Verification items for the finished model (mm, model axes). A direction names the side the tool comes from. Coordinates: 2 decimals unless noted, no trailing zeros. Order: outer loops, then holes, each group sorted by start corner. A loop starts at its lowest first (then second) coordinate and runs counter-clockwise, first axis right, second up.
Q1. Set-up check for faces 1 (the flat face through (63.3, 50.6, 1.6)), 2 (the flat face through (49.9, 62.6, 1.6)), 3 (the flat face through (-62.6, 49.9, 1.6)): record each of +Z, -Z, +X, -X, +Y, -Y from which the full face is reachable in a straight line by a thin tool's end or side.
Q2. Depth check by flat-ended pin: P1, Ø1.5, axis at x = 65, z = 2, coming from the +Y side; P2, Ø1.5, axis at x = -42, z = 2, coming from the -Y side; P3, Ø1, axis at y = -24.5, z = 2.5, coming from the -X side. Enter the tip coordinate at first touch or a pass-through.
Q3. Cross-section at B-B, the plane y = 51.5. Record the boundary of the cut face in (x, z) (3 decimals), and give its area (3 significant figures).
Q4. Draft check along Y on faces 4 (the flat face through (-49.9, -62.6, 1.6)), 5 (the cylindrical face through (-0.419, 28.484, 1.565)), 6 (the flat face through (62.6, -49.9, 1.6)). Enter one of: pulls with the +Y half, pulls with the -Y half, needs draft (parallel to the pull), parting line crosses it, or undercut.
Q5. Cross-section at A-A, the plane x = -69. Record the boundary of the cut face in (y, z) (3 decimals), and give its area (3 significant figures).
Q6. Cross-section at D-D, the plane y = 12. Record the boundary of the cut face in (x, z) (3 decimals).
Q7. Thickness scan on line 1 (X direction, y = 59, z = 1.7); line 2 (Y direction, x = 74, z = 2.5); line 3 (X direction, y = -53.5, z = 1.85). Record the ranges inside material, lowest first.
from build123d import *

# Parameters (mm, degrees)
F0_W     = 177.8
F0_H     = 177.8
F1_DEPTH = 3.175
F3_DEPTH = 3.176
F4_R     = 38.1
F5_R     = 8.89


# Not quite as in the source:
# - a length typed as a fraction of an inch, garbled in the dataset ("3 / 203.2 mm" for 3/8 in), is restored


with BuildPart() as f1:
    # F0 (on Top) → F1 (new body)
    with BuildSketch(Plane.XY):
        Rectangle(F0_W, F0_H)
    extrude(amount=F1_DEPTH)

    # F2 (on face) → F3 (cut, through all)
    with BuildSketch(Plane.XY.offset(3.175)):
        Polygon((76.2, 88.9), (-76.2, 88.9), (0, 12.7), align=None)
        Polygon((88.9, -76.2), (88.9, 76.2), (12.7, 0), align=None)
        Polygon((-76.2, -88.9), (76.2, -88.9), (0, -12.7), align=None)
        Polygon((-12.7, 0), (-88.9, 76.2), (-88.9, -76.2), align=None)
    extrude(amount=-F3_DEPTH, mode=Mode.SUBTRACT)

    # F4
    f4_edges = [f1.edges().sort_by_distance(p)[0] for p in [
        (0, -12.7, 1.5875),
        (12.7, 0, 1.5875),
        (0, 12.7, 1.5875),
        (-12.7, 0, 1.5875),
    ]]
    fillet(f4_edges, radius=F4_R)

    # F5
    f5_edges = [f1.edges().sort_by_distance(p)[0] for p in [
        (88.9, 88.9, 1.5875),
        (88.9, 76.2, 1.5875),
        (88.9, -76.2, 1.5875),
        (88.9, -88.9, 1.5875),
        (76.2, -88.9, 1.5875),
        (-76.2, -88.9, 1.5875),
        (-88.9, -88.9, 1.5875),
        (-88.9, -76.2, 1.5875),
        (-88.9, 76.2, 1.5875),
        (-88.9, 88.9, 1.5875),
        (-76.2, 88.9, 1.5875),
        (76.2, 88.9, 1.5875),
    ]]
    fillet(f5_edges, radius=F5_R)


solid = f1.part
Check values:
1. face 1: +Z, -Z, +X
1. face 2: +Z, -Z, +Y
1. face 3: +Z, -Z, -X
2. P1: stops at y = 78.45
2. P2: stops at y = -55.45
2. P3: stops at x = -37.83
3. outline: (-64.2, 0) - (-38.8, 0) - (-38.8, 3.175) - (-64.2, 3.175) - close; (38.8, 0) - (64.2, 0) - (64.2, 3.175) - (38.8, 3.175) - close
3. area: 161 mm2
4. face 4: pulls with the -Y half
4. face 5: pulls with the +Y half
4. face 6: undercut
5. outline: (-81.7, 0) - (-56.3, 0) - (-56.3, 3.175) - (-81.7, 3.175) - close; (56.3, 0) - (81.7, 0) - (81.7, 3.175) - (56.3, 3.175) - close
5. area: 161 mm2
6. outline: (-30.421, 0) - (30.421, 0) - (30.421, 3.175) - (-30.421, 3.175) - close
7. line 1: x = -71.7 to -46.3, 46.3 to 71.7
7. line 2: y = -86.68 to -61.3, 61.3 to 86.68
7. line 3: x = -66.2 to -40.8, 40.8 to 66.2
